```python
from build123d import *

# Parameters (mm, degrees)
SKETCH2_R           = 9
SKETCH2_R_2         = 6
BOSS_EXTRUDE1_DEPTH = 20
SKETCH3_R           = 6
BOSS_EXTRUDE2_DEPTH = 5
FILLET1_R           = 2
CUT_EXTRUDE1_REACH  = 7
SKETCH4_R           = 1.6
CHAMFER1_SIZE       = 5
FILLET2_R           = 4
CHAMFER2_SIZE       = 1.2


with BuildPart() as part:
    # Sketch2 → Boss-Extrude1 (new body)
    with BuildSketch(Plane.XY):
        with Locations((-135, -82.312657819)):
            Circle(SKETCH2_R)
        with Locations((-135, -82.312657819)):
            Circle(SKETCH2_R_2, mode=Mode.SUBTRACT)
    extrude(amount=BOSS_EXTRUDE1_DEPTH)

    # Sketch3 → Boss-Extrude2 (add)
    with BuildSketch(Plane(origin=(0, 0, 0), x_dir=(-1, 0, 0), z_dir=(0, 0, -1))):
        with BuildLine():
            Line((152, -102.312657819), (118, -102.312657819))
            ThreePointArc((118, -102.312657819), (115.878679656, -101.433978162), (115, -99.312657819))
            Line((115, -99.312657819), (115, -65.312657819))
            ThreePointArc((115, -65.312657819), (115.878679656, -63.191337475), (118, -62.312657819))
            Line((118, -62.312657819), (152, -62.312657819))
            ThreePointArc((152, -62.312657819), (154.121320344, -63.191337475), (155, -65.312657819))
            Line((155, -65.312657819), (155, -99.312657819))
            ThreePointArc((155, -99.312657819), (154.121320344, -101.433978162), (152, -102.312657819))
        make_face()
        with Locations((135, -82.312657819)):
            Circle(SKETCH3_R, mode=Mode.SUBTRACT)
    extrude(amount=-BOSS_EXTRUDE2_DEPTH)

    # Fillet1
    fillet1_edges = [part.edges().sort_by_distance(p)[0] for p in [
        (-115.878679656, -101.433978162, 5),
        (-115, -82.312657819, 5),
        (-115.878679656, -63.191337475, 5),
        (-135, -62.312657819, 5),
        (-154.121320344, -63.191337475, 5),
        (-155, -82.312657819, 5),
        (-154.121320344, -101.433978162, 5),
        (-135, -102.312657819, 5),
    ]]
    fillet(fillet1_edges, radius=FILLET1_R)

    # Sketch4 → Cut-Extrude1 (cut, up to next)
    with BuildSketch(Plane.XY.offset(5), mode=Mode.PRIVATE) as cut_extrude1_sk1:
        with Locations((-150, -67.312657819)):
            Circle(SKETCH4_R)
    cut_extrude1_tool1 = extrude(cut_extrude1_sk1.sketch, amount=-CUT_EXTRUDE1_REACH, mode=Mode.PRIVATE) & part.part
    add(cut_extrude1_tool1.solids().sort_by_distance((-150, -67.312658, 5))[0], mode=Mode.SUBTRACT)
    # Sketch4 → Cut-Extrude1 (cut, up to next)
    with BuildSketch(Plane.XY.offset(5), mode=Mode.PRIVATE) as cut_extrude1_sk2:
        with Locations((-120, -67.312657819)):
            Circle(SKETCH4_R)
    cut_extrude1_tool2 = extrude(cut_extrude1_sk2.sketch, amount=-CUT_EXTRUDE1_REACH, mode=Mode.PRIVATE) & part.part
    add(cut_extrude1_tool2.solids().sort_by_distance((-120, -67.312658, 5))[0], mode=Mode.SUBTRACT)
    # Sketch4 → Cut-Extrude1 (cut, up to next)
    with BuildSketch(Plane.XY.offset(5), mode=Mode.PRIVATE) as cut_extrude1_sk3:
        with Locations((-120, -97.312657819)):
            Circle(SKETCH4_R)
    cut_extrude1_tool3 = extrude(cut_extrude1_sk3.sketch, amount=-CUT_EXTRUDE1_REACH, mode=Mode.PRIVATE) & part.part
    add(cut_extrude1_tool3.solids().sort_by_distance((-120, -97.312658, 5))[0], mode=Mode.SUBTRACT)
    # Sketch4 → Cut-Extrude1 (cut, up to next)
    with BuildSketch(Plane.XY.offset(5), mode=Mode.PRIVATE) as cut_extrude1_sk4:
        with Locations((-150, -97.312657819)):
            Circle(SKETCH4_R)
    cut_extrude1_tool4 = extrude(cut_extrude1_sk4.sketch, amount=-CUT_EXTRUDE1_REACH, mode=Mode.PRIVATE) & part.part
    add(cut_extrude1_tool4.solids().sort_by_distance((-150, -97.312658, 5))[0], mode=Mode.SUBTRACT)

    # Chamfer1
    chamfer1_edges = [part.edges().sort_by_distance(p)[0] for p in [
        (-144, -82.312657819, 5),
    ]]
    chamfer(chamfer1_edges, length=CHAMFER1_SIZE)

    # Fillet2
    fillet2_edges = [part.edges().sort_by_distance(p)[0] for p in [
        (-144, -82.312657819, 10),
        (-149, -82.312657819, 5),
    ]]
    fillet(fillet2_edges, radius=FILLET2_R)

    # Chamfer2
    chamfer2_edges = [part.edges().sort_by_distance(p)[0] for p in [
        (-151.6, -97.312657819, 5),
        (-121.6, -97.312657819, 5),
        (-121.6, -67.312657819, 5),
        (-151.6, -67.312657819, 5),
    ]]
    chamfer(chamfer2_edges, length=CHAMFER2_SIZE)


solid = part.part
```
Input: part model. Units: mm. Frame: model coordinates. Coordinates: 2 decimals unless noted, no trailing zeros. Loops run counter-clockwise (first coordinate to the right, second up) from the corner with the lowest first, then second, coordinate; pieces in that order, holes last.
Q1. Contact query for flat-ended pins moving along their axis: pin 1 (3.5 mm diameter, centred on x = -150, y = -97.31, fed in from +Z); pin 2 (4 mm diameter, centred on y = -72.5, z = 5.5, fed in from -X); pin 3 (4 mm diameter, centred on y = -88.5, z = 11, fed in from +X). Output: stop coordinate, or through.
Results are:
pin 1: stops at z = 3.95
pin 2: stops at x = -154.94
pin 3: stops at x = -126.68
Q2. Mould query, pull axis Y, two halves, no side actions, for faces 1 (the conical face through (-142.592, -89.274, 8.699)), 2 (the cylindrical face through (-139.422, -78.258, 9.86)), 3 (the flat face through (-115, -83, 1)), 4 (the cylindrical face through (-115.86, -63.21, 1.48)). Classes: +Y half, -Y half, draft (parallel to the pull), parting line (faces both ways), or undercut.
Results are:
face 1: parting line
face 2: undercut
face 3: draft
face 4: +Y half
Q3. Section B-B, the plane z = 18.25. Return the cut outline in (x, y), and give its area (3 significant figures).
Results are:
outline: circle Ø18 at (-135, -82.31); hole circle Ø12 at (-135, -82.31)
area: 141 mm2
Q4. Line query: line 1 along Y through (x, z) = (-120, 2); line 2 along Z through (x, y) = (-126, -69); line 3 along X through (y, z) = (-85.5, 12). Output: solid intervals per line, ascending.
Results are:
line 1: y = -102.31 to -98.91, -95.71 to -68.91, -65.71 to -62.31
line 2: z = 0 to 5
line 3: x = -143.42 to -140.08, -129.92 to -126.58
Q5. Section A-A, the plane x = -150. Give the number of separate pieces and of enclosed holes in the cut face, and give its area (3 significant figures).
Results are:
separate pieces: 3
enclosed holes: 0
area: 164 mm2
